Design review of the part shown in the three views and the two pictorial views. Dimensions are in mm from the part's minimum x, y and z. Give positions to 0.01 mm unless a question says otherwise; leave off trailing zeros. Write each loop counter-clockwise with the first axis right and the second up, starting at its lowest first coordinate (ties: lowest second). Pieces come first, ordered by that corner, then holes. Notation, with made-up numbers: (44, 89) -> (58, 89) arc R20 cw to (58, 119) -> close; hole circle Ø1 at (43, -4.5). An arc over 180 degrees is marked (long way). Return JSON: item names as keys, results as strings. Group by question number.
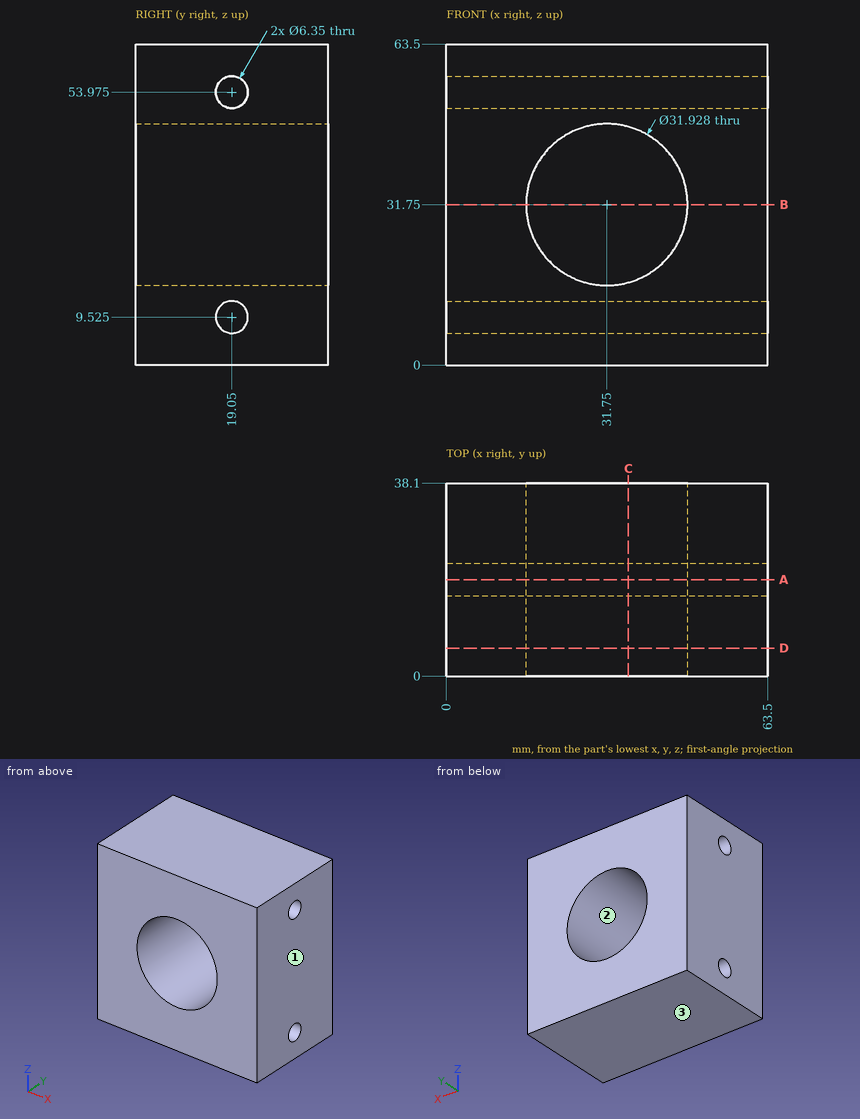
Q1. For L1, parallel to Z at x = 35, y = 17; L2, parallel to Z at x = 14, y = 19; L3, parallel to Z at x = 18, y = 19.05, list the stretches that pass through material, from the lowest coordinate up. Write a range as from..to.
Q2. Insertion check: pin 1 (12 mm diameter, centred on x = 45.5, z = 26.5, fed in from -Y); pin 2 (6 mm diameter, centred on x = 35, z = 42, fed in from +Y). Each pin has a flat end and moves straight along its axis. Give the tip position at first contact, or say it passes through.
Q3. Take a section at B-B, the plane z = 31.75. Give the boundary of the cut face in (x, y).
Q4. Take a section at C-C, the plane x = 36. Count the separate pieces of the cut face and the enclosed holes in it, plus the area to 3 significant figures.
Q5. Mouldability with a two-part tool opening along X and no side actions: class the marked faces 1, 2 and 3 as +X half, -X half, draft (parallel to the pull), parting line (faces both ways), or undercut.
Q6. Take a section at D-D, the plane y = 5.5. Give the boundary of the cut face in (x, z), plus the area to 3 significant figures.
Q7. Take a section at A-A, the plane y = 19.05. Give the boundary of the cut face in (x, z), plus the area to 4 significant figures.
Final values:
{
 "1": {"L1": "z = 0..7.1, 11.95..16.12, 47.38..51.55, 56.4..63.5", "L2": "z = 0..6.35, 12.7..50.8, 57.15..63.5", "L3": "z = 0..6.35, 12.7..23.64, 39.86..50.8, 57.15..63.5"},
 "2": {"pin 1": "stops at y = 0", "pin 2": "passes through"},
 "3": {"outline": "(0, 0) -> (15.79, 0) -> (15.79, 38.1) -> (0, 38.1) -> close; (47.71, 0) -> (63.5, 0) -> (63.5, 38.1) -> (47.71, 38.1) -> close"},
 "4": {"separate pieces": "2", "enclosed holes": "2", "area": "1,180 mm²"},
 "5": {"face 1": "+X half", "face 2": "undercut", "face 3": "draft"},
 "6": {"outline": "(0, 0) -> (63.5, 0) -> (63.5, 63.5) -> (0, 63.5) -> close; hole circle Ø31.93 at (31.75, 31.75)", "area": "3,230 mm²"},
 "7": {"outline": "(0, 0) -> (63.5, 0) -> (63.5, 6.35) -> (0, 6.35) -> close; (0, 12.7) -> (63.5, 12.7) -> (63.5, 50.8) -> (0, 50.8) -> close; (0, 57.15) -> (63.5, 57.15) -> (63.5, 63.5) -> (0, 63.5) -> close; hole circle Ø31.93 at (31.75, 31.75)", "area": "2,425 mm²"}
}
